from build123d import *

# Parameters (mm, degrees)
ESQUISSE1_W             = 15
ESQUISSE1_H             = 15
BOSS_EXTRU_1_DEPTH      = 11.5
ESQUISSE2_W             = 12
ESQUISSE2_H             = 15
ENL_V_MAT_EXTRU_1_DEPTH = 10
CONG_1_R                = 2
ESQUISSE3_W             = 0.5
ESQUISSE3_H             = 6
BOSS_EXTRU_2_DEPTH      = 0.5
ENL_V_MAT_EXTRU_2_DEPTH = 6
ESQUISSE5_W             = 3.5
ESQUISSE5_H             = 4
ESQUISSE5_H_2           = 2
BOSS_EXTRU_3_DEPTH      = 0.4
ESQUISSE6_W             = 0.4
ESQUISSE6_H             = 4
ESQUISSE6_H_2           = 2
BOSS_EXTRU_4_DEPTH      = 3.1
CONG_3_R                = 0.5
ESQUISSE7_W             = 6.75
ESQUISSE7_H             = 10.5
BOSS_EXTRU_5_DEPTH      = 1.5
ESQUISSE12_R            = 1.25
ENL_V_MAT_EXTRU_6_DEPTH = 1.5
BOSS_EXTRU_6_DEPTH      = 4.25
ENL_V_MAT_EXTRU_7_DEPTH = 10.5
CONG_5_R                = 2
CHANFREIN2_SIZE         = 0.25
CHANFREIN3_SIZE         = 0.25
CHANFREIN4_SIZE         = 0.25


with BuildPart() as part:
    # Esquisse1 → Boss.-Extru.1 (new body)
    with BuildSketch(Plane.XY):
        Rectangle(ESQUISSE1_W, ESQUISSE1_H)
    extrude(amount=BOSS_EXTRU_1_DEPTH)

    # Esquisse2 → Enlèv. mat.-Extru.1 (cut)
    with BuildSketch(Plane(origin=(0, 0, 0), x_dir=(-1, 0, 0), z_dir=(0, 0, -1))):
        Rectangle(ESQUISSE2_W, ESQUISSE2_H)
    extrude(amount=-ENL_V_MAT_EXTRU_1_DEPTH, mode=Mode.SUBTRACT)

    # Congé1
    cong_1_edges = [part.edges().sort_by_distance(p)[0] for p in [
        (-7.5, 0, 11.5),
        (7.5, 0, 11.5),
    ]]
    fillet(cong_1_edges, radius=CONG_1_R)

    # Esquisse3 → Boss.-Extru.2 (add)
    with BuildSketch(Plane(origin=(0, 0, 10), x_dir=(-1, 0, 0), z_dir=(0, 0, -1))):
        with Locations((-5.75, 4.5)):
            Rectangle(ESQUISSE3_W, ESQUISSE3_H)
        with Locations((5.75, 4.5)):
            Rectangle(ESQUISSE3_W, ESQUISSE3_H)
    extrude(amount=BOSS_EXTRU_2_DEPTH)

    # Esquisse4 → Enlèv. mat.-Extru.2 (cut)
    with BuildSketch(Plane.XZ.offset(-1.5)):
        with BuildLine():
            Line((-6, 9.5), (-5.5, 9.5))
            Line((-5.5, 9.5), (-5.5, 10))
            ThreePointArc((-5.5, 10), (-5.853553391, 9.853553391), (-6, 9.5))
        make_face()
        with BuildLine():
            Line((6, 9.5), (5.5, 9.5))
            Line((5.5, 9.5), (5.5, 10))
            ThreePointArc((5.5, 10), (5.853553391, 9.853553391), (6, 9.5))
        make_face()
    extrude(amount=-ENL_V_MAT_EXTRU_2_DEPTH, mode=Mode.SUBTRACT)

    # Esquisse5 → Boss.-Extru.3 (add)
    with BuildSketch(Plane(origin=(0, 0, 10), x_dir=(-1, 0, 0), z_dir=(0, 0, -1))):
        with Locations((-4.25, -4.5)):
            Rectangle(ESQUISSE5_W, ESQUISSE5_H)
        with Locations((-4.25, -0.5)):
            Rectangle(ESQUISSE5_W, ESQUISSE5_H_2)
    extrude(amount=BOSS_EXTRU_3_DEPTH)

    # Esquisse6 → Boss.-Extru.4 (add)
    with BuildSketch(Plane(origin=(0, 0, 9.6), x_dir=(-1, 0, 0), z_dir=(0, 0, -1))):
        with Locations((-5.8, -4.5)):
            Rectangle(ESQUISSE6_W, ESQUISSE6_H)
        with Locations((-5.8, -0.5)):
            Rectangle(ESQUISSE6_W, ESQUISSE6_H_2)
    extrude(amount=BOSS_EXTRU_4_DEPTH)

    # Congé3
    cong_3_edges = [part.edges().sort_by_distance(p)[0] for p in [
        (5.6, -4.5, 9.6),
        (5.6, -0.5, 9.6),
    ]]
    fillet(cong_3_edges, radius=CONG_3_R)

    # Esquisse7 → Boss.-Extru.5 (add)
    with BuildSketch(Plane(origin=(0, 0, 0), x_dir=(-1, 0, 0), z_dir=(0, 0, -1))):
        with Locations((-10.875, -2.25)):
            Rectangle(ESQUISSE7_W, ESQUISSE7_H)
        with Locations((10.875, -2.25)):
            Rectangle(ESQUISSE7_W, ESQUISSE7_H)
    extrude(amount=-BOSS_EXTRU_5_DEPTH)

    # Esquisse12 → Enlèv. mat.-Extru.6 (cut)
    with BuildSketch(Plane(origin=(0, 0, 0), x_dir=(-1, 0, 0), z_dir=(0, 0, -1))):
        with Locations((10.75, -2.25)):
            Circle(ESQUISSE12_R)
        with Locations((-10.75, -2.25)):
            Circle(ESQUISSE12_R)
    extrude(amount=-ENL_V_MAT_EXTRU_6_DEPTH, mode=Mode.SUBTRACT)

    # Esquisse13 → Boss.-Extru.6 (add)
    with BuildSketch(Plane.XY.offset(1.5)):
        Polygon((-7.5, 3), (-7.5, -7.5), (-14.25, -7.5), (-14.25, -3.342912687), (-13.107019699, -3.342912687), (-10.75, -4.703738644), (-8.625, -3.476869322), (-8.625, -1.023130678), (-10.75, 0.203738644), (-13.107019699, -1.157087313), (-14.25, -1.157087313), (-14.25, 3), align=None)
        Polygon((7.5, -7.5), (7.5, 3), (14.25, 3), (14.25, -1.023130678), (12.875, -1.023130678), (10.75, 0.203738644), (8.625, -1.023130678), (8.625, -3.476869322), (10.75, -4.703738644), (12.875, -3.476869322), (14.25, -3.476869322), (14.25, -7.5), align=None)
    extrude(amount=BOSS_EXTRU_6_DEPTH)

    # Esquisse14 → Enlèv. mat.-Extru.7 (cut)
    with BuildSketch(Plane.XZ.offset(7.5)):
        Polygon((-7.5, 5.75), (-14.25, 1.5), (-14.25, 5.75), align=None)
        Polygon((7.5, 5.75), (14.25, 1.5), (14.25, 5.75), align=None)
    extrude(amount=-ENL_V_MAT_EXTRU_7_DEPTH, mode=Mode.SUBTRACT)

    # Congé5
    cong_5_edges = [part.edges().sort_by_distance(p)[0] for p in [
        (-14.25, -7.5, 0.75),
        (-14.25, 3, 0.75),
        (14.25, 3, 0.75),
        (14.25, -7.5, 0.75),
    ]]
    fillet(cong_5_edges, radius=CONG_5_R)

    # Chanfrein2
    chanfrein2_edges = [part.edges().sort_by_distance(p)[0] for p in [
        (-11.928509849, -4.023325665, 2.961678984),
        (-9.6875, -4.090303983, 4.372685185),
        (-8.625, -2.25, 5.041666667),
        (-9.6875, -0.409696017, 4.372685185),
        (-11.928509849, -0.476674335, 2.961678984),
        (11.8125, -0.409696017, 3.034722222),
        (9.6875, -0.409696017, 4.372685185),
        (8.625, -2.25, 5.041666667),
        (9.6875, -4.090303983, 4.372685185),
        (11.8125, -4.090303983, 3.034722222),
    ]]
    chamfer(chanfrein2_edges, length=CHANFREIN2_SIZE)

    # Chanfrein3
    chanfrein3_edges = [part.edges().sort_by_distance(p)[0] for p in [
        (-9.5, -2.25, 0),
        (12, -2.25, 0),
    ]]
    chamfer(chanfrein3_edges, length=CHANFREIN3_SIZE)

    # Chanfrein4
    chanfrein4_edges = [part.edges().sort_by_distance(p)[0] for p in [
        (3.8, 0.5, 9.6),
        (5.6, -6.5, 7.8),
        (5.6, -2.5, 7.8),
        (5.6, -1.5, 7.8),
        (5.6, 0.5, 7.8),
        (3.8, -1.5, 9.6),
        (3.8, -6.5, 9.6),
        (5.453553391, 0.5, 9.453553391),
        (5.453553391, -1.5, 9.453553391),
        (5.453553391, -2.5, 9.453553391),
        (5.453553391, -6.5, 9.453553391),
        (3.8, -2.5, 9.6),
    ]]
    chamfer(chanfrein4_edges, length=CHANFREIN4_SIZE)


solid = part.part
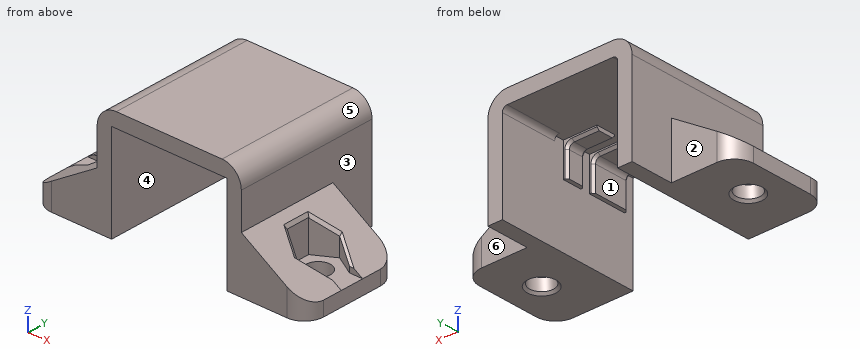
CAD build for the part. Positions are in the model's coordinates, mm. Face numbers are marked on the shaded views. A direction names the side the tool comes from. Round coordinates to 2 decimals unless told otherwise and drop trailing zeros. Order: outer loops, then holes, each group sorted by start corner. A loop starts at its lowest first (then second) coordinate and runs counter-clockwise, first axis right, second up. Notation, with made-up numbers: (58, -17) - (94, -17) arc R28 ccw to (94, 13) - close; hole circle Ø3 at (89, 4.5). An arc over 180 degrees is marked (long way). Return JSON: item names as keys, results as strings.
(1) Wall check: probe 1 along X at (y, z) = (3.75, 8.75); probe 2 along Y at (x, z) = (10.75, 0.7); probe 3 along Z at (x, y) = (-4.5, 6). Give the ranges that are in metal, low to high. Write a range as from..to.
Answer key:
{"probe 1": "x = -7.5..-6, 6..7.5", "probe 2": "y = -7.5..-3.5, -1..3", "probe 3": "z = 10..11.5"}
(2) Cut at A-A (z = 8.5). Give the cut face in (x, y).
Answer key:
{"outline": "(-7.5, -7.5) - (-6, -7.5) - (-6, 7.5) - (-7.5, 7.5) - close; (5.6, -6.25) - (5.85, -6.5) - (6, -6.5) - (6, -7.5) - (7.5, -7.5) - (7.5, 7.5) - (6, 7.5) - (6, 0.5) - (5.85, 0.5) - (5.6, 0.25) - (5.6, -1.25) - (5.85, -1.5) - (6, -1.5) - (6, -2.5) - (5.85, -2.5) - (5.6, -2.75) - close"}
(3) Cut at B-B (y = 6.75). Give the cut face in (x, z), then the cut area to 3 significant figures.
Answer key:
{"outline": "(-7.5, 0) - (-6, 0) - (-6, 9.5) arc R0.5 cw to (-5.5, 10) - (5.5, 10) arc R0.5 cw to (6, 9.5) - (6, 0) - (7.5, 0) - (7.5, 9.5) arc R2 ccw to (5.5, 11.5) - (-5.5, 11.5) arc R2 ccw to (-7.5, 9.5) - close", "area": "50.9 mm^2"}
(4) Cut at D-D (x = -3.75). Give the cut face in (y, z).
Answer key:
{"outline": "(-7.5, 10) - (7.5, 10) - (7.5, 11.5) - (-7.5, 11.5) - close"}
(5) Pin check, flat tips, straight feed: pin 1 Ø0.8 at (y, z) = (-2, 3.5) entering from -X (3 decimals); pin 2 Ø5.5 at (x, y) = (10.5, -3) entering from +Z; pin 3 Ø2 at (y, z) = (-4, 8) entering from -X. Stop position of each tip, or through.
Answer key:
{"pin 1": "stops at x = -8.625", "pin 2": "stops at z = 5.59", "pin 3": "stops at x = -7.5"}
(6) Tool access for the marked faces 1, 2 and 3: list every direction of +Z, -Z, +X, -X, +Y, -Y with a clear straight run to the whole face (end or side of a thin tool).
Answer key:
{"face 1": "-Z, +Y, -Y", "face 2": "+Z, -Z, -X, +Y", "face 3": "+Z, +X, +Y"}
(7) Cut at C-C (x = 4.75). Give the cut face in (y, z).
Answer key:
{"outline": "(-7.5, 10) - (-6.5, 10) - (-6.5, 9.85) - (-6.25, 9.6) - (-2.75, 9.6) - (-2.5, 9.85) - (-2.5, 10) - (-1.5, 10) - (-1.5, 9.85) - (-1.25, 9.6) - (0.25, 9.6) - (0.5, 9.85) - (0.5, 10) - (7.5, 10) - (7.5, 11.5) - (-7.5, 11.5) - close"}
(8) Pull direction X, two halves, no side cores. Call the marked faces 4, 5 and 6: +X half, -X half, draft (parallel to the pull), parting line (faces both ways), or undercut.
Answer key:
{"face 4": "undercut", "face 5": "+X half", "face 6": "draft"}
